from build123d import *

# Parameters (mm, degrees)
SKETCH1_W                = 126.7
SKETCH1_H                = 14
BRACKETBASE_DEPTH        = 5
SKETCH2_R                = 1.375
MOUNTINGHOLES_DEPTH      = 1
MOUNTINGHOLES_DEPTH_BACK = 6
SKETCH5_W                = 126.7
SKETCH5_H                = 8.25
BASEEXTENSION_DEPTH      = 5
REVOLVE1_ANGLE           = 180
REVOLVE2_ANGLE           = 180
REVOLVE3_ANGLE           = 180
REVOLVE4_ANGLE           = 180
SKETCH9_W                = 15
SKETCH9_H                = 5
CUT_EXTRUDE2_DEPTH       = 4.25
CUT_EXTRUDE2_DEPTH_BACK  = 6
CUT_EXTRUDE3_DEPTH       = 4.25
CUT_EXTRUDE3_DEPTH_BACK  = 6
SKETCH11_R               = 2.5
CUT_EXTRUDE4_DEPTH       = 23.25
SKETCH12_R               = 2.5
CUT_EXTRUDE5_DEPTH       = 23.25
SKETCH13_W               = 6.5
SKETCH13_H               = 5
CUT_EXTRUDE6_DEPTH       = 1.0000001
CUT_EXTRUDE6_DEPTH_BACK  = 23.25
BOSS_EXTRUDE1_DEPTH      = 1


with BuildPart() as part:
    # Sketch1 → bracketBase (new body)
    with BuildSketch(Plane.XY):
        with Locations((63.35, 7)):
            Rectangle(SKETCH1_W, SKETCH1_H)
    extrude(amount=BRACKETBASE_DEPTH)

    # Sketch2 → mountingHoles (cut, two sides)
    with BuildSketch(Plane.XY.offset(5)) as mountingholes_sk:
        with Locations((63.35, 10)):
            Circle(SKETCH2_R)
        with Locations((63.35, 3)):
            Circle(SKETCH2_R)
        with Locations((123.7, 10)):
            Circle(SKETCH2_R)
        with Locations((123.7, 3)):
            Circle(SKETCH2_R)
        with Locations((3, 3)):
            Circle(SKETCH2_R)
        with Locations((3, 10)):
            Circle(SKETCH2_R)
    extrude(amount=MOUNTINGHOLES_DEPTH, mode=Mode.SUBTRACT)
    extrude(mountingholes_sk.sketch, amount=-MOUNTINGHOLES_DEPTH_BACK, mode=Mode.SUBTRACT)

    # Sketch5 → baseExtension (add)
    with BuildSketch(Plane.XY.offset(5)):
        with Locations((63.35, 18.125)):
            Rectangle(SKETCH5_W, SKETCH5_H)
    extrude(amount=-BASEEXTENSION_DEPTH)

    # Sketch4 → Revolve1 (revolve)
    with BuildSketch(Plane.XY.offset(5)):
        with BuildLine():
            Line((43.425, 9.00715266), (43.425, 15.50715266))
            ThreePointArc((43.425, 15.50715266), (40.175, 12.25715266), (43.425, 9.00715266))
        make_face()
    revolve(axis=Axis((43.425, 9.00715266, 5), (0, 1, 0)), revolution_arc=REVOLVE1_ANGLE)

    # Sketch6 → Revolve2 (revolve)
    with BuildSketch(Plane.XY.offset(5)):
        with BuildLine():
            Line((22.925, 9.00715266), (22.925, 15.50715266))
            ThreePointArc((22.925, 15.50715266), (26.175, 12.25715266), (22.925, 9.00715266))
        make_face()
    revolve(axis=Axis((22.925, 9.00715266, 5), (0, -1, 0)), revolution_arc=REVOLVE2_ANGLE)

    # Sketch7 → Revolve3 (revolve)
    with BuildSketch(Plane.XY.offset(5)):
        with BuildLine():
            Line((83.275, 9.00715266), (83.275, 15.50715266))
            ThreePointArc((83.275, 15.50715266), (86.525, 12.25715266), (83.275, 9.00715266))
        make_face()
    revolve(axis=Axis((83.275, 9.00715266, 5), (0, -1, 0)), revolution_arc=REVOLVE3_ANGLE)

    # Sketch8 → Revolve4 (revolve)
    with BuildSketch(Plane.XY.offset(5)):
        with BuildLine():
            Line((103.775, 9.00715266), (103.775, 15.50715266))
            ThreePointArc((103.775, 15.50715266), (100.525, 12.25715266), (103.775, 9.00715266))
        make_face()
    revolve(axis=Axis((103.775, 9.00715266, 5), (0, 1, 0)), revolution_arc=REVOLVE4_ANGLE)

    # Sketch9 → Cut-Extrude2 (cut, two sides)
    with BuildSketch(Plane.XY.offset(5)) as cut_extrude2_sk:
        with Locations((33.175, 19.75)):
            Rectangle(SKETCH9_W, SKETCH9_H)
        with Locations((93.525, 19.75)):
            Rectangle(SKETCH9_W, SKETCH9_H)
    extrude(amount=CUT_EXTRUDE2_DEPTH, mode=Mode.SUBTRACT)
    extrude(cut_extrude2_sk.sketch, amount=-CUT_EXTRUDE2_DEPTH_BACK, mode=Mode.SUBTRACT)

    # Sketch10 → Cut-Extrude3 (cut, two sides)
    with BuildSketch(Plane.XY.offset(5)) as cut_extrude3_sk:
        Polygon((116.025, 22.25), (126.7, 14), (126.7, 22.25), align=None)
        Polygon((0, 14), (0, 22.25), (10.675, 22.25), align=None)
    extrude(amount=CUT_EXTRUDE3_DEPTH, mode=Mode.SUBTRACT)
    extrude(cut_extrude3_sk.sketch, amount=-CUT_EXTRUDE3_DEPTH_BACK, mode=Mode.SUBTRACT)

    # Sketch11 → Cut-Extrude4 (cut, through all)
    with BuildSketch(Plane.XZ):
        with Locations((126.95, 1.155770847)):
            Circle(SKETCH11_R)
        with Locations((-0.25, 1.155770847)):
            Circle(SKETCH11_R)
    extrude(amount=-CUT_EXTRUDE4_DEPTH, mode=Mode.SUBTRACT)

    # Sketch12 → Cut-Extrude5 (cut, through all)
    with BuildSketch(Plane.XZ):
        with Locations((117.7, 0)):
            Circle(SKETCH12_R)
        with Locations((73.7, 0)):
            Circle(SKETCH12_R)
        with Locations((53, 0)):
            Circle(SKETCH12_R)
        with Locations((9, 0)):
            Circle(SKETCH12_R)
    extrude(amount=-CUT_EXTRUDE5_DEPTH, mode=Mode.SUBTRACT)

    # Sketch13 → Cut-Extrude6 (cut, two sides)
    with BuildSketch(Plane.XZ) as cut_extrude6_sk:
        with Locations((123.45, 2.5)):
            Rectangle(SKETCH13_W, SKETCH13_H)
        with Locations((3.25, 2.5)):
            Rectangle(SKETCH13_W, SKETCH13_H)
    extrude(amount=CUT_EXTRUDE6_DEPTH, mode=Mode.SUBTRACT)
    extrude(cut_extrude6_sk.sketch, amount=-CUT_EXTRUDE6_DEPTH_BACK, mode=Mode.SUBTRACT)

    # Sketch14 → Boss-Extrude1 (add)
    with BuildSketch(Plane.XZ):
        with BuildLine():
            Line((120.2, 0), (120.2, 5))
            Line((120.2, 5), (6.5, 5))
            Line((6.5, 5), (6.5, 0))
            ThreePointArc((6.5, 0), (9, 2.5), (11.5, 0))
            Line((11.5, 0), (50.5, 0))
            ThreePointArc((50.5, 0), (53, 2.5), (55.5, 0))
            Line((55.5, 0), (71.2, 0))
            ThreePointArc((71.2, 0), (73.7, 2.5), (76.2, 0))
            Line((76.2, 0), (115.2, 0))
            ThreePointArc((115.2, 0), (117.7, 2.5), (120.2, 0))
        make_face()
    extrude(amount=BOSS_EXTRUDE1_DEPTH)


solid = part.part
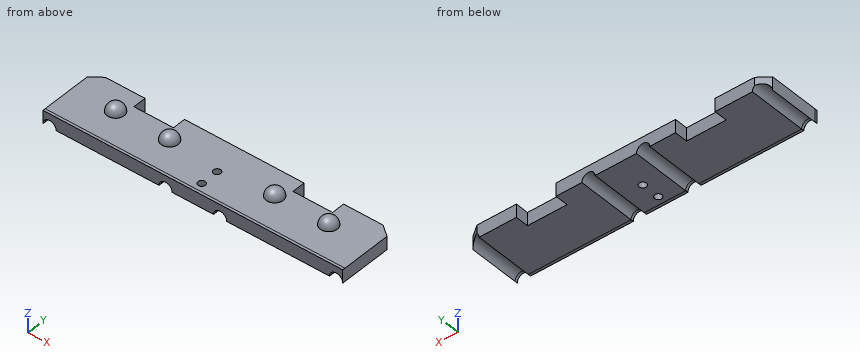
Model file for the job. Use its own axes, mm. Round coordinates to 2 decimals unless told otherwise and drop trailing zeros. Loops run counter-clockwise (first coordinate to the right, second up) from the corner with the lowest first, then second, coordinate; pieces in that order, holes last.
1. Drop flat-ended pins along their axis: P1, Ø3, axis at x = 102.5, y = 6, coming from the +Z side; P2, Ø1.5, axis at y = 20, z = 2.5, coming from the +X side; P3, Ø1.5, axis at x = 91, z = 3.5, coming from the +Y side. Give the stop position or say it passes through.
Check values:
P1: stops at z = 5
P2: stops at x = 119.91
P3: stops at y = 17.25
2. Band-saw the part on C-C, the plane z = 3.5. List the corners of the cut face in (x, y) (3 decimals).
Check values:
outline: (6.5, -1) - (120.2, -1) - (120.2, 19.023) - (116.025, 22.25) - (101.025, 22.25) - (101.025, 17.25) - (86.025, 17.25) - (86.025, 22.25) - (40.675, 22.25) - (40.675, 17.25) - (25.675, 17.25) - (25.675, 22.25) - (10.675, 22.25) - (6.5, 19.023) - close; hole circle Ø2.75 at (63.35, 3); hole circle Ø2.75 at (63.35, 10)
3. Wall check: probe 1 along X at (y, z) = (19, 3.5) (3 decimals); probe 2 along Y at (x, z) = (63.35, 2.05) (3 decimals); probe 3 along Z at (x, y) = (30, 6.5). Give the ranges that are in metal, low to high.
Check values:
probe 1: x = 6.5 to 25.675, 40.675 to 86.025, 101.025 to 120.2
probe 2: y = -1 to 1.625, 4.375 to 8.625, 11.375 to 22.25
probe 3: z = 0 to 5
4. Band-saw the part on A-A, the plane y = 3. List the corners of the cut face in (x, z) (3 decimals), and give its area (3 significant figures).
Check values:
outline: (6.5, 0) arc R2.5 cw to (11.5, 0) - (50.5, 0) arc R2.5 cw to (55.5, 0) - (61.975, 0) - (61.975, 5) - (6.5, 5) - close; (64.725, 0) - (71.2, 0) arc R2.5 cw to (76.2, 0) - (115.2, 0) arc R2.5 cw to (120.2, 0) - (120.2, 5) - (64.725, 5) - close
area: 515 mm2
5. Band-saw the part on B-B, the plane x = 63.35. List the corners of the cut face in (y, z) (3 decimals).
Check values:
outline: (-1, 0) - (1.625, 0) - (1.625, 5) - (-1, 5) - close; (4.375, 0) - (8.625, 0) - (8.625, 5) - (4.375, 5) - close; (11.375, 0) - (22.25, 0) - (22.25, 5) - (11.375, 5) - close
6. Band-saw the part on D-D, the plane x = 84.5. List the corners of the cut face in (y, z).
Check values:
outline: (-1, 0) - (22.25, 0) - (22.25, 5) - (15.27, 5) arc R3.01 ccw to (9.25, 5) - (-1, 5) - close
